```python
from build123d import *

# Parameters (mm, degrees)
SKETCH_R     = 10
SKETCH_R_2   = 2
PAD_DEPTH    = 10
CHAMFER_SIZE = 1


with BuildPart() as part:
    # Sketch → Pad (new body)
    with BuildSketch(Plane.XZ):
        Circle(SKETCH_R)
        Circle(SKETCH_R_2, mode=Mode.SUBTRACT)
    extrude(amount=PAD_DEPTH)

    # Chamfer
    chamfer_edges = [part.edges().sort_by_distance(p)[0] for p in [
        (-2, -10, 0),
        (-2, 0, 0),
        (-10, -10, 0),
        (-10, 0, 0),
    ]]
    chamfer(chamfer_edges, length=CHAMFER_SIZE)


solid = part.part
```
Work out the finished part from the listing and answer in its coordinate system (mm). Coordinates: 2 decimals unless noted, no trailing zeros. Order: outer loops, then holes, each group sorted by start corner. A loop starts at its lowest first (then second) coordinate and runs counter-clockwise, first axis right, second up. Notation, with made-up numbers: M -32,53.25 L -26,53.25 A26 cw -26,72.25 Z; hole C 9,70 d1. An arc over 180 degrees is marked long. Use CSV: the item, a comma, the result in double quotes.
1) Section C-C on y = -7.25 is taken. Write down the section's boundary in (x, z).
Worked out:
outline,"C 0,0 d20; hole C 0,0 d4"
2) Consider line 1 (Z direction, x = 0, y = -6); line 2 (X direction, y = -9.5, z = 2.75); line 3 (X direction, y = -2.75, z = -8). Determine where each line is inside the solid, lowest interval first. Write a range as [from, to].
Worked out:
line 1,"z = [-10, -2], [2, 10]"
line 2,"x = [-9.09, 9.09]"
line 3,"x = [-6, 6]"
3) Determine the mould class of faces 1 (the face through (-2.17, -4.94, -9.76)), 2 (the face through (0, -5, -2)), 3 (the face through (0, 0, -4)) for opening direction X: released by +X, released by -X, zero draft, split by the parting line, or undercut.
Worked out:
face 1,"split by the parting line"
face 2,"undercut"
face 3,"zero draft"
4) Flat-ended cylindrical pins translate along their axes: pin 1 Ø5 at (x, y) = (-8, -6.5) entering from +Z; pin 2 Ø1 at (x, y) = (5.5, -9) entering from -Z; pin 3 Ø2 at (y, z) = (-1.5, 7) entering from +X. Find the tip coordinate at first contact, or state that the pin passes through.
Worked out:
pin 1,"stops at z = 8.35"
pin 2,"stops at z = -8.66"
pin 3,"stops at x = 8"
5) Section A-A on x = 0 is taken. Write down the section's boundary in (y, z).
Worked out:
outline,"M -10,-9 L -9,-10 L -1,-10 L 0,-9 L 0,-3 L -1,-2 L -9,-2 L -10,-3 Z; M -10,3 L -9,2 L -1,2 L 0,3 L 0,9 L -1,10 L -9,10 L -10,9 Z"
6) Section B-B on z = 0 is taken. Write down the section's boundary in (x, y), plus the area to 3 significant figures.
Worked out:
outline,"M -10,-9 L -9,-10 L -3,-10 L -2,-9 L -2,-1 L -3,0 L -9,0 L -10,-1 Z; M 2,-9 L 3,-10 L 9,-10 L 10,-9 L 10,-1 L 9,0 L 3,0 L 2,-1 Z"
area,"156 mm^2"
